Here's how the part is built. I have some questions about the finished solid (model axes, mm). Coordinates: 2 decimals unless noted, no trailing zeros. Write each loop counter-clockwise with the first axis right and the second up, starting at its lowest first coordinate (ties: lowest second). Pieces come first, ordered by that corner, then holes.
```python
from build123d import *

# Parameters (mm, degrees)
BOSS_EXTRUDE1_DEPTH      = 35
BOSS_EXTRUDE1_DEPTH_BACK = 35
SKETCH1_W                = 32
SKETCH1_H                = 2
SKETCH2_R                = 2
CUT_EXTRUDE2_DEPTH       = 2
SKETCH3_R                = 2
CUT_EXTRUDE3_DEPTH       = 2


with BuildPart() as part:
    # Sketch1 → Boss-Extrude1 (new, two sides: drawn at the far end of the back side and taken through both)
    with BuildSketch(Plane(origin=(0, 0, 0), x_dir=(0, 0, -1), z_dir=(1, 0, 0)).offset(-BOSS_EXTRUDE1_DEPTH_BACK)):
        with Locations((0, 1)):
            Rectangle(SKETCH1_W, SKETCH1_H)
    extrude(amount=BOSS_EXTRUDE1_DEPTH + BOSS_EXTRUDE1_DEPTH_BACK)

    # Sketch2 → Cut-Extrude2 (cut)
    with BuildSketch(Plane(origin=(0, 2, 0), x_dir=(1, 0, 0), z_dir=(0, 1, 0))):
        with Locations(Location((-23.335, 0, 0), (0, 0, 270))):
            Circle(SKETCH2_R)
        with Locations(Location((23.335, 0, 0), (0, 0, 270))):
            Circle(SKETCH2_R)
    extrude(amount=-CUT_EXTRUDE2_DEPTH, mode=Mode.SUBTRACT)

    # Sketch3 → Cut-Extrude3 (cut)
    with BuildSketch(Plane(origin=(0, 2, 0), x_dir=(1, 0, 0), z_dir=(0, 1, 0))):
        with Locations(Location((0, 10, 0), (0, 0, 270))):
            Circle(SKETCH3_R)
        with Locations(Location((0, 2, 0), (0, 0, 270))):
            Circle(SKETCH3_R)
        with Locations(Location((0, -7.12, 0), (0, 0, 270))):
            Circle(SKETCH3_R)
    extrude(amount=-CUT_EXTRUDE3_DEPTH, mode=Mode.SUBTRACT)


solid = part.part
```
1) Imagine slicing it at C-C on y = 1.2. Please give me the cut outline in (x, z) (3 decimals).
Values follow:
outline: (-35, -16) - (35, -16) - (35, 16) - (-35, 16) - close; hole circle Ø4 at (-23.335, 0); hole circle Ø4 at (0, -10); hole circle Ø4 at (0, -2); hole circle Ø4 at (0, 7.12); hole circle Ø4 at (23.335, 0)
2) I need wall thicknesses on probe 1 along Z at (x, y) = (-1.5, 0.6); probe 2 along X at (y, z) = (0.4, -10); probe 3 along X at (y, z) = (1.2, 0.5). Which ranges of each line are inside material? Lowest first, please.
Values follow:
probe 1: z = -16 to -11.32, -8.68 to -3.32, -0.68 to 5.8, 8.44 to 16
probe 2: x = -35 to -2, 2 to 35
probe 3: x = -35 to -25.27, -21.4 to 21.4, 25.27 to 35
3) Imagine slicing it at B-B on x = 0. Please give me the cut outline in (y, z), then the cut area to 3 significant figures.
Values follow:
outline: (0, -16) - (2, -16) - (2, -12) - (0, -12) - close; (0, -8) - (2, -8) - (2, -4) - (0, -4) - close; (0, 0) - (2, 0) - (2, 5.12) - (0, 5.12) - close; (0, 9.12) - (2, 9.12) - (2, 16) - (0, 16) - close
area: 40.0 mm2
4) Imagine slicing it at A-A on z = 7.12. Please give me the cut outline in (x, y).
Values follow:
outline: (-35, 0) - (-2, 0) - (-2, 2) - (-35, 2) - close; (2, 0) - (35, 0) - (35, 2) - (2, 2) - close
5) Will these pins go through, and if not, where does the flat tip stop? pin 1 (3.5 mm diameter, centred on x = 0, z = -2, fed in from +Y); pin 2 (1.5 mm diameter, centred on x = 25, z = -10.5, fed in from -Y).
Values follow:
pin 1: passes through
pin 2: stops at y = 0
